Input: part model. Units: mm. Frame: model coordinates. Face numbers are marked on the shaded views. Round coordinates to 2 decimals unless told otherwise and drop trailing zeros. Order: outer loops, then holes, each group sorted by start corner. A loop starts at its lowest first (then second) coordinate and runs counter-clockwise, first axis right, second up. Notation, with made-up numbers: (79, 75) - (113, 75) arc R12 ccw to (113, 82) - close; hole circle Ø8 at (54, -25.75). An arc over 180 degrees is marked (long way). One line per item, written item: value. Start each with the question number.
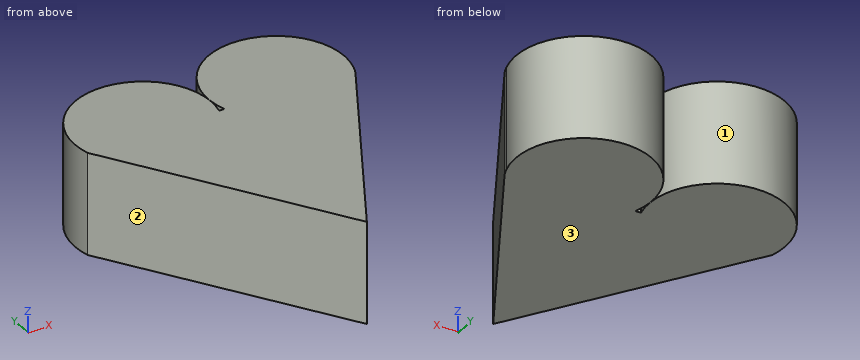
from build123d import *

# Parameters (mm, degrees)
F1_DEPTH = 38.1


with BuildPart() as f1:
    # F0 (on Top) → F1 (new body)
    with BuildSketch(Plane.XY):
        with BuildLine():
            Line((-59.369042, 37.685493), (-61.37024, 37.685493))
            ThreePointArc((-61.37024, 37.685493), (-85.964896, 69.4308), (-110.559551, 37.685493))
            Line((-110.559551, 37.685493), (-57.076961, -44.962659))
            Line((-57.076961, -44.962659), (-12.102065, 34.814507))
            ThreePointArc((-12.102065, 34.814507), (-11.501003, 36.233084), (-10.987052, 37.685493))
            ThreePointArc((-10.987052, 37.685493), (-35.178047, 70.828604), (-59.369042, 37.685493))
        make_face()
    extrude(amount=F1_DEPTH)


solid = f1.part
Item 1: Section query C-C on x = -39. Return loops of the section in (y, z), and give its area (3 significant figures).
Item 2: First-contact query: pin 1 Ø8 at (y, z) = (18.5, 17.5) entering from -X; pin 2 Ø8 at (x, z) = (-28, 15) entering from +Y; pin 3 Ø8 at (y, z) = (36, 25) entering from +X. Flat tips, straight axial feed; report the tip coordinate or a pass-through.
Item 3: Section query A-A on z = 19. Return loops of the section in (x, y), and give its area (3 significant figures).
Item 4: Line query: L1, parallel to X at y = 61.5, z = 15; L2, parallel to X at y = 58.5, z = 28; L3, parallel to X at y = 33.5, z = 28.5. Output: solid intervals per line, ascending.
Item 5: Pull-direction query (X, two-part tool) for the marked faces 1, 2 and 3; classes: released by +X, released by -X, zero draft, split by the parting line, or undercut.
Item 6: Section query B-B on y = 62.5. Return loops of the section in (x, z), and give its area (3 significant figures).
Item 7: Section query D-D on y = 24. Return loops of the section in (x, z), and give its area (3 significant figures).
Geometry results:
1. outline: (-12.9, 0) - (70.54, 0) - (70.54, 38.1) - (-12.9, 38.1) - close
1. area: 3,180 mm^2
2. pin 1: stops at x = -100.73
2. pin 2: stops at y = 70.63
2. pin 3: stops at x = -10.36
3. outline: (-110.56, 37.69) - (-57.08, -44.96) - (-12.1, 34.81) arc R25.4 ccw to (-10.99, 37.69) arc R25.4 ccw (long way) to (-59.37, 37.69) - (-61.37, 37.69) arc R25.4 ccw (long way) to start
3. area: 6,870 mm^2
4. L1: x = -104.4 to -67.53, -54.85 to -15.51
4. L2: x = -106.84 to -65.09, -56.96 to -13.4
4. L3: x = -107.85 to -12.84
5. face 1: undercut
5. face 2: released by -X
5. face 3: zero draft
6. outline: (-103.4, 0) - (-68.53, 0) - (-68.53, 38.1) - (-103.4, 38.1) - close; (-53.99, 0) - (-16.37, 0) - (-16.37, 38.1) - (-53.99, 38.1) - close
6. area: 2,760 mm^2
7. outline: (-101.7, 0) - (-18.2, 0) - (-18.2, 38.1) - (-101.7, 38.1) - close
7. area: 3,180 mm^2
